Check sheet for the modelled part. Datum: model origin and axes. Units: mm. Face numbers are marked on the shaded views. Give positions to 0.01 mm unless a question says otherwise; leave off trailing zeros. Loops run counter-clockwise (first coordinate to the right, second up) from the corner with the lowest first, then second, coordinate; pieces in that order, holes last. Notation, with made-up numbers: (86.25, 6) - (112.25, 6) arc R29 ccw to (112.25, 30) - close; hole circle Ø10 at (70.5, 61.5). An arc over 180 degrees is marked (long way). Answer in a Markdown table with one row per item. Add a question column.
(1) Thickness scan on L1, parallel to X at y = -3.5, z = 0; L2, parallel to X at y = -5, z = 0; L3, parallel to X at y = -2.75, z = -6.25. Record the ranges inside material, lowest first.
(2) Sectioned sample at C-C on z = -6. Enter the section's corners in (x, y).
(3) Draft check along X on the marked faces 1 and 2. Enter one of: released by +X, released by -X, zero draft, split by the parting line, or undercut.
(4) Sectioned sample at D-D on x = 44. Enter the section's corners in (y, z) (1 decimal).
(5) Sectioned sample at B-B on y = 2.25. Enter the section's corners in (x, z).
(6) Go/stop test with flat-tipped pins: P1, Ø4, axis at x = -37.5, z = 2.5, coming from the +Y side; P2, Ø5, axis at x = 51, z = -5, coming from the +Y side; P3, Ø5, axis at x = 11, y = -5, coming from the -Z side. Record where each tip stops, or that it passes through.
(7) Sectioned sample at A-A on z = 0. Enter the section's corners in (x, y).
from build123d import *

# Parameters (mm, degrees)
SKETCH1_R           = 7.9375
BOSS_EXTRUDE1_DEPTH = 76.581
SKETCH3_R           = 3.96875
BOSS_EXTRUDE2_DEPTH = 6.35
SKETCH4_R           = 3.96875
BOSS_EXTRUDE3_DEPTH = 6.35
SKETCH2_W           = 82.532989992
SKETCH2_H           = 25.4
CUT_EXTRUDE1_DEPTH  = 8.9375
SKETCH5_R           = 1.7272
CUT_EXTRUDE2_DEPTH  = 8.9375


with BuildPart() as part:
    # Sketch1 → Boss-Extrude1 (new body, symmetric)
    with BuildSketch(Plane(origin=(0, 0, 0), x_dir=(0, 0, -1), z_dir=(1, 0, 0))):
        Circle(SKETCH1_R)
    extrude(amount=BOSS_EXTRUDE1_DEPTH, both=True)

    # Sketch3 → Boss-Extrude2 (add)
    with BuildSketch(Plane.ZY.offset(76.581)):
        Circle(SKETCH3_R)
    extrude(amount=BOSS_EXTRUDE2_DEPTH)

    # Sketch4 → Boss-Extrude3 (add)
    with BuildSketch(Plane(origin=(76.581, 0, 0), x_dir=(0, 0, -1), z_dir=(1, 0, 0))):
        Circle(SKETCH4_R)
    extrude(amount=BOSS_EXTRUDE3_DEPTH)

    # Sketch2 → Cut-Extrude1 (cut, through all)
    with BuildSketch(Plane(origin=(0, 0, 0), x_dir=(1, 0, 0), z_dir=(0, 1, 0))):
        with Locations((-8.279380004, 0)):
            Rectangle(SKETCH2_W, SKETCH2_H)
    extrude(amount=CUT_EXTRUDE1_DEPTH, mode=Mode.SUBTRACT)

    # Sketch5 → Cut-Extrude2 (cut, through all)
    with BuildSketch(Plane(origin=(0, 0, 0), x_dir=(1, 0, 0), z_dir=(0, 1, 0))):
        with Locations((-40.719375, 0)):
            Circle(SKETCH5_R)
        with Locations((-8.279380004, 0)):
            Circle(SKETCH5_R)
        with Locations((24.160614992, 0)):
            Circle(SKETCH5_R)
    extrude(amount=-CUT_EXTRUDE2_DEPTH, mode=Mode.SUBTRACT)


solid = part.part
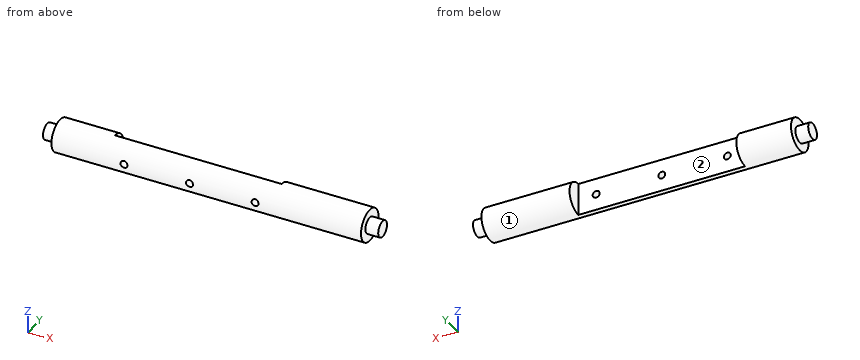
Reply:
| question | item | result |
|---|---|---|
| 1 | L1 | -82.93 to -42.45, -38.99 to -10.01, -6.55 to 22.43, 25.89 to 82.93 |
| 1 | L2 | -76.58 to -42.45, -38.99 to -10.01, -6.55 to 22.43, 25.89 to 76.58 |
| 1 | L3 | -76.58 to 76.58 |
| 2 | outline | (-76.58, -5.2) - (76.58, -5.2) - (76.58, 5.2) - (32.99, 5.2) - (32.99, 0) - (-49.55, 0) - (-49.55, 5.2) - (-76.58, 5.2) - close |
| 3 | face 1 | zero draft |
| 3 | face 2 | undercut |
| 4 | outline | circle Ø15.9 at (0, 0) |
| 5 | outline | (-82.93, -3.27) - (-76.58, -3.27) - (-76.58, -7.61) - (-49.55, -7.61) - (-49.55, 7.61) - (-76.58, 7.61) - (-76.58, 3.27) - (-82.93, 3.27) - close; (32.99, -7.61) - (76.58, -7.61) - (76.58, -3.27) - (82.93, -3.27) - (82.93, 3.27) - (76.58, 3.27) - (76.58, 7.61) - (32.99, 7.61) - close |
| 6 | P1 | y = 0 |
| 6 | P2 | y = 7.53 |
| 6 | P3 | z = -7.53 |
| 7 | outline | (-82.93, -3.97) - (-76.58, -3.97) - (-76.58, -7.94) - (-42.45, -7.94) - (-42.45, 0) - (-49.55, 0) - (-49.55, 7.94) - (-76.58, 7.94) - (-76.58, 3.97) - (-82.93, 3.97) - close; (-38.99, -7.94) - (-10.01, -7.94) - (-10.01, 0) - (-38.99, 0) - close; (-6.55, -7.94) - (22.43, -7.94) - (22.43, 0) - (-6.55, 0) - close; (25.89, -7.94) - (76.58, -7.94) - (76.58, -3.97) - (82.93, -3.97) - (82.93, 3.97) - (76.58, 3.97) - (76.58, 7.94) - (32.99, 7.94) - (32.99, 0) - (25.89, 0) - close |
